Build history of the part. All positions in model axes, mm. Give positions to 0.01 mm unless a question says otherwise; leave off trailing zeros. Order: outer loops, then holes, each group sorted by start corner. A loop starts at its lowest first (then second) coordinate and runs counter-clockwise, first axis right, second up. Notation, with made-up numbers: M 66.5,-30 L 101.5,-30 A35 ccw 101.5,9 Z; hole C 27.5,-22.5 d6. An arc over 180 degrees is marked long. Use CSV: the item, a comma, the result in double quotes. Start each with the question number.
Item 1: Band-saw the part on B-B on z = -6. Write the cut outline in (x, y).
Item 2: Band-saw the part on A-A on x = 0. Write the cut outline in (y, z).
Item 3: Wall check: line 1 along X through (y, z) = (3.45, 0); line 2 along X through (y, z) = (4.6, 9.5). Give the ranges that are in metal, low to high.
Item 4: Pin check, flat tips, straight feed: P1, Ø2, axis at y = 3.5, z = -5.5, coming from the -X side; P2, Ø2.5, axis at x = 20.5, y = 3, coming from the +Z side; P3, Ø1.5, axis at x = -16.5, y = 3.5, coming from the +Z side; P4, Ø8, axis at x = -28, z = 24.5, coming from the -Y side. Stop position of each tip, or through.
Item 5: Band-saw the part on C-C on y = 2.5. Give the number of separate pieces and of enclosed holes in the cut face, plus the area to 3 significant figures.
Item 6: Band-saw the part on D-D on z = 18.5. Write the cut outline in (x, y).
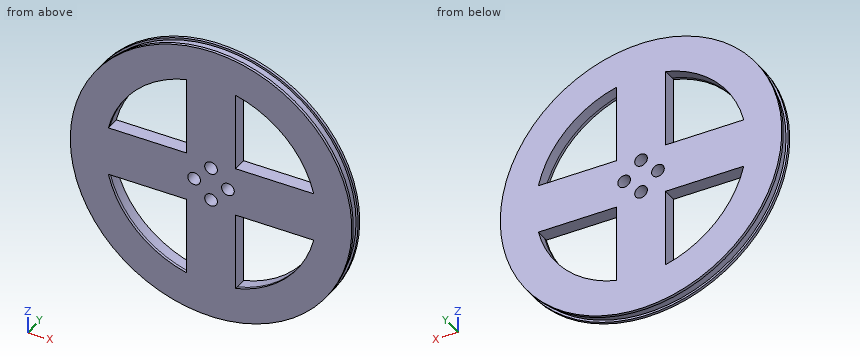
Autodesk Inventor part; units mm, degrees
ref_plane "YZ Plane" through (0, 0, 0) normal (1, 0, 0) x (0, 1, 0)
ref_plane "XZ Plane" through (0, 0, 0) normal (0, 1, 0) x (-1, 0, 0)
ref_plane "XY Plane" through (0, 0, 0) normal (0, 0, 1) x (1, 0, 0)
sketch "Sketch1" plane through (0, 0, 0) normal (0, 1, 0) x (-1, 0, 0)
  circle A0 centre (0, 0) radius 50
  circle A1 centre (0, 0) radius 37.5
  circle A2 centre (0, 0) radius 8.75
  line L0 (37.5, 0) -> (42.141, 0) construction
  line L1 (8.75, -8.75) -> (36.4649, -8.75)
  line L2 (-8.75, -8.75) -> (-36.4649, -8.75)
  line L3 (-8.75, -8.75) -> (-8.75, -36.4649)
  line L4 (8.75, -8.75) -> (8.75, -36.4649)
  line L5 (8.75, 8.75) -> (36.4649, 8.75)
  line L6 (-8.75, 8.75) -> (-36.4649, 8.75)
  line L7 (-8.75, 8.75) -> (-8.75, 36.4649)
  line L8 (8.75, 8.75) -> (8.75, 36.4649)
  dimension "d1" = 75
  dimension "d0" = 100
  dimension "d2" = 17.5
extrude "Extrusion1" add sketch "Sketch1" along normal blind 1 contours A0 | A1 L1 L4 L3 L2 L6 L7 L8 L5 | A2
sketch "Sketch6" plane through (0, 1, 0) normal (0, 1, 0) x (1, 0, 0)
  circle A0 centre (0, 0) radius 49.25
  line L0 (-36.4649, -8.75) -> (-8.75, -8.75)
  line L1 (-8.6444, -8.75) -> (-36.4649, -8.75)
  arc A1 (-36.4649, -8.75) -> (-8.75, -36.4649) centre (0, 0) ccw
  line L2 (-36.4649, -8.75) -> (-36.4649, -8.75)
  line L3 (-8.75, -36.4649) -> (-8.75, -8.75)
  line L4 (-8.75, -8.75) -> (-8.75, -36.4649)
  arc A2 (-36.4649, -8.75) -> (-8.75, -36.4649) centre (0, 0) ccw
  line L5 (0, 0) -> (0, -21.0072)
  line L6 (0, 0) -> (-15.0352, 0)
  line L7 (36.4649, -8.75) -> (8.75, -8.75)
  arc A3 (8.75, -36.4649) -> (36.4649, -8.75) centre (0, 0) ccw
  line L8 (8.75, -36.4649) -> (8.75, -8.75)
  line L9 (-36.4649, 8.75) -> (-8.75, 8.75)
  arc A4 (-8.75, 36.4649) -> (-36.4649, 8.75) centre (0, 0) ccw
  line L10 (-8.75, 36.4649) -> (-8.75, 8.75)
  arc A5 (36.4649, 8.75) -> (8.75, 36.4649) centre (0, 0) ccw
  line L11 (36.4649, 8.75) -> (8.75, 8.75)
  line L12 (8.75, 36.4649) -> (8.75, 8.75)
  dimension "d33" = 98.5
extrude "Extrusion3" add sketch "Sketch6" along normal blind 3
sketch "Sketch7" plane through (0, 4, 0) normal (0, 1, 0) x (1, 0, 0)
  circle A0 centre (0, 0) radius 50
  line L0 (-8.75, -36.4649) -> (-8.75, -8.75)
  arc A1 (-36.4649, -8.75) -> (-8.75, -36.4649) centre (0, 0) ccw
  line L1 (-8.75, -8.75) -> (-36.4649, -8.75)
  line L2 (-8.75, -8.75) -> (-8.75, -36.4649)
  arc A2 (-36.4649, -8.75) -> (-8.75, -36.4649) centre (0, 0) ccw
  line L3 (0, 0) -> (0, -13.8921)
  line L4 (0, 0) -> (-12.1262, 0)
  line L5 (8.75, -36.4649) -> (8.75, -8.75)
  arc A3 (8.75, -36.4649) -> (36.4649, -8.75) centre (0, 0) ccw
  line L6 (8.75, -8.75) -> (36.4649, -8.75)
  line L7 (-8.75, 36.4649) -> (-8.75, 8.75)
  arc A4 (-8.75, 36.4649) -> (-36.4649, 8.75) centre (0, 0) ccw
  line L8 (-8.75, 8.75) -> (-36.4649, 8.75)
  line L9 (8.75, 8.75) -> (36.4649, 8.75)
  arc A5 (36.4649, 8.75) -> (8.75, 36.4649) centre (0, 0) ccw
  line L10 (8.75, 36.4649) -> (8.75, 8.75)
  dimension "d37" = 100
extrude "Extrusion4" add sketch "Sketch7" along normal blind 1
sketch "Sketch8" plane through (0, 5, 0) normal (0, 1, 0) x (1, 0, 0)
  circle A0 centre (0, 6) radius 2.25
  line L0 (0, 0) -> (-6, 0)
  line L1 (0, 0) -> (0, -5.6539)
  circle A1 centre (0, -6) radius 2.25
  circle A2 centre (-6, 0) radius 2.25
  circle A3 centre (6, 0) radius 2.25
  dimension "d40" = 4.5
  dimension "d41" = 6
  dimension "d42" = 4.5
  dimension "d43" = 6
hole "Hole2" at (0, 5, 6) at (-6, 5, 0) at (0, 5, -6) at (6, 5, 0) direction (0, -1, 0) diameter 4.5 end through all
properties part number "wheel"
Model answer:
1,outline,"M -49.64,0 L -2.25,0 L -2.25,5 L -49.64,5 L -49.64,4 L -48.88,4 L -48.88,1 L -49.64,1 Z; M 2.25,0 L 49.64,0 L 49.64,1 L 48.88,1 L 48.88,4 L 49.64,4 L 49.64,5 L 2.25,5 Z"
2,outline,"M 0,-50 L 1,-50 L 1,-49.25 L 4,-49.25 L 4,-50 L 5,-50 L 5,-8.25 L 0,-8.25 Z; M 0,-3.75 L 5,-3.75 L 5,3.75 L 0,3.75 Z; M 0,8.25 L 5,8.25 L 5,50 L 4,50 L 4,49.25 L 1,49.25 L 1,50 L 0,50 Z"
3,line 1,"x = -49.25 to -8.25, -3.75 to 3.75, 8.25 to 49.25"
3,line 2,"x = -49.09 to -36.28, -8.75 to 8.75, 36.28 to 49.09"
4,P1,"stops at x = -49.78"
4,P2,"stops at z = 45.93"
4,P3,"stops at z = 47.39"
4,P4,"stops at y = 0"
5,separate pieces,"1"
5,enclosed holes,"8"
5,area,"5,430 mm^2"
6,outline,"M -46.45,0 L -32.62,0 L -32.62,5 L -46.45,5 L -46.45,4 L -45.64,4 L -45.64,1 L -46.45,1 Z; M -8.75,0 L 8.75,0 L 8.75,5 L -8.75,5 Z; M 32.62,0 L 46.45,0 L 46.45,1 L 45.64,1 L 45.64,4 L 46.45,4 L 46.45,5 L 32.62,5 Z"
